```python
from build123d import *

# Parameters (mm, degrees)
SKETCH1_W             = 54
SKETCH1_H             = 54
BOSS_EXTRUDE1_DEPTH   = 10
CUT_EXTRUDE2_DEPTH    = 40.471508712
CUT_EXTRUDE3_DEPTH    = 2
SKETCH4_R             = 13.75
CUT_EXTRUDE4_DEPTH    = 1
SKETCH5_W             = 2
SKETCH5_H             = 10
SKETCH5_W_2           = 10
SKETCH5_H_2           = 2
CUT_EXTRUDE5_DEPTH    = 4
SKETCH7_R             = 8.75
CUT_EXTRUDE7_DEPTH    = 0.5
CROQUIS1_W            = 54
CROQUIS1_H            = 54
CORTAR_EXTRUIR1_DEPTH = 4


with BuildPart() as part:
    # Sketch1 → Boss-Extrude1 (new body)
    with BuildSketch(Plane(origin=(0, 0, 0), x_dir=(1, 0, 0), z_dir=(0, 1, 0))):
        Rectangle(SKETCH1_W, SKETCH1_H)
    extrude(amount=BOSS_EXTRUDE1_DEPTH)

    # Sketch2 → Cut-Extrude2 (cut, through all)
    with BuildSketch(Plane(origin=(0, 10, 0), x_dir=(1, 0, 0), z_dir=(0, 1, 0))):
        with BuildLine():
            ThreePointArc((-17, -14), (-16.121320344, -16.121320344), (-14, -17))
            Line((-14, -17), (-2, -17))
            Line((-2, -17), (-2, -14.866068747))
            ThreePointArc((-2, -14.866068747), (-10.606601718, -10.606601718), (-14.866068747, -2))
            Line((-14.866068747, -2), (-17, -2))
            Line((-17, -2), (-17, -14))
        make_face()
        with BuildLine():
            Line((2, -14.866068747), (2, -17))
            Line((2, -17), (14, -17))
            ThreePointArc((14, -17), (16.121320344, -16.121320344), (17, -14))
            Line((17, -14), (17, -2))
            Line((17, -2), (14.866068747, -2))
            ThreePointArc((14.866068747, -2), (10.606601718, -10.606601718), (2, -14.866068747))
        make_face()
        with BuildLine():
            Line((-17, 14), (-17, 2))
            Line((-17, 2), (-14.866068747, 2))
            ThreePointArc((-14.866068747, 2), (-10.606601718, 10.606601718), (-2, 14.866068747))
            Line((-2, 14.866068747), (-2, 17))
            Line((-2, 17), (-14, 17))
            ThreePointArc((-14, 17), (-16.121320344, 16.121320344), (-17, 14))
        make_face()
        with BuildLine():
            Line((14.866068747, 2), (17, 2))
            Line((17, 2), (17, 14))
            ThreePointArc((17, 14), (16.121320344, 16.121320344), (14, 17))
            Line((14, 17), (2, 17))
            Line((2, 17), (2, 14.866068747))
            ThreePointArc((2, 14.866068747), (10.606601718, 10.606601718), (14.866068747, 2))
        make_face()
    extrude(amount=-CUT_EXTRUDE2_DEPTH, mode=Mode.SUBTRACT)

    # Sketch3 → Cut-Extrude3 (cut)
    with BuildSketch(Plane(origin=(0, 10, 0), x_dir=(1, 0, 0), z_dir=(0, 1, 0))):
        with BuildLine():
            Line((-14, -17), (14, -17))
            ThreePointArc((14, -17), (16.121320344, -16.121320344), (17, -14))
            Line((17, -14), (17, 14))
            ThreePointArc((17, 14), (16.121320344, 16.121320344), (14, 17))
            Line((14, 17), (-14, 17))
            ThreePointArc((-14, 17), (-16.121320344, 16.121320344), (-17, 14))
            Line((-17, 14), (-17, -14))
            ThreePointArc((-17, -14), (-16.121320344, -16.121320344), (-14, -17))
        make_face()
    extrude(amount=-CUT_EXTRUDE3_DEPTH, mode=Mode.SUBTRACT)

    # Sketch4 → Cut-Extrude4 (cut)
    with BuildSketch(Plane(origin=(0, 8, 0), x_dir=(1, 0, 0), z_dir=(0, 1, 0))):
        with Locations(Location((0, 0, 0), (0, 0, 270))):
            Circle(SKETCH4_R)
    extrude(amount=-CUT_EXTRUDE4_DEPTH, mode=Mode.SUBTRACT)

    # Sketch5 → Cut-Extrude5 (cut)
    with BuildSketch(Plane(origin=(0, 10, 0), x_dir=(1, 0, 0), z_dir=(0, 1, 0))):
        with Locations((0, -22)):
            Rectangle(SKETCH5_W, SKETCH5_H)
        with BuildLine():
            Line((1, -17), (1, -13.713588152))
            ThreePointArc((1, -13.713588152), (0, -13.75), (-1, -13.713588152))
            Line((-1, -13.713588152), (-1, -17))
            Line((-1, -17), (1, -17))
        make_face()
        with Locations((22, 0)):
            Rectangle(SKETCH5_W_2, SKETCH5_H_2)
        with BuildLine():
            Line((17, 1), (13.713588152, 1))
            ThreePointArc((13.713588152, 1), (13.75, 0), (13.713588152, -1))
            Line((13.713588152, -1), (17, -1))
            Line((17, -1), (17, 1))
        make_face()
        with BuildLine():
            Line((1, 17), (-1, 17))
            Line((-1, 17), (-1, 13.713588152))
            ThreePointArc((-1, 13.713588152), (0, 13.75), (1, 13.713588152))
            Line((1, 13.713588152), (1, 17))
        make_face()
        with Locations((0, 22)):
            Rectangle(SKETCH5_W, SKETCH5_H)
        with Locations((-22, 0)):
            Rectangle(SKETCH5_W_2, SKETCH5_H_2)
        with BuildLine():
            Line((-13.713588152, 1), (-17, 1))
            Line((-17, 1), (-17, -1))
            Line((-17, -1), (-13.713588152, -1))
            ThreePointArc((-13.713588152, -1), (-13.75, 0), (-13.713588152, 1))
        make_face()
    extrude(amount=-CUT_EXTRUDE5_DEPTH, mode=Mode.SUBTRACT)

    # Sketch7 → Cut-Extrude7 (cut)
    with BuildSketch(Plane(origin=(0, 7, 0), x_dir=(1, 0, 0), z_dir=(0, 1, 0))):
        with Locations(Location((0, 0, 0), (0, 0, 270))):
            Circle(SKETCH7_R)
    extrude(amount=-CUT_EXTRUDE7_DEPTH, mode=Mode.SUBTRACT)

    # Croquis1 → Cortar-Extruir1 (cut)
    with BuildSketch(Plane.XZ):
        Rectangle(CROQUIS1_W, CROQUIS1_H)
    extrude(amount=-CORTAR_EXTRUIR1_DEPTH, mode=Mode.SUBTRACT)


solid = part.part
```
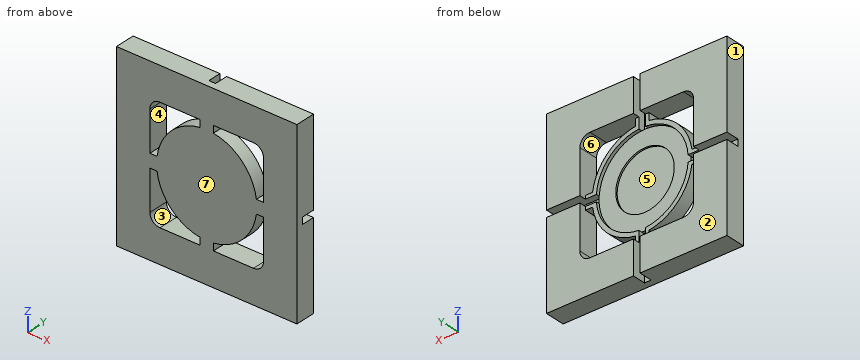
Build history of the part. All positions in model axes, mm. Face numbers are marked on the shaded views. A direction names the side the tool comes from. Round coordinates to 2 decimals unless told otherwise and drop trailing zeros. Order: outer loops, then holes, each group sorted by start corner. A loop starts at its lowest first (then second) coordinate and runs counter-clockwise, first axis right, second up. Notation, with made-up numbers: (-14.75, 40) -> (24.25, 40) arc R18 ccw to (24.25, 54) -> close; hole circle Ø7 at (47.25, -17.5). An arc over 180 degrees is marked (long way). Answer in a Markdown table with one row per item.
1) Mould opens along X. For the marked faces 1, 2, 3 and 4 say: released by +X, released by -X, zero draft, split by the parting line, or undercut.
Values:
| item | result |
|---|---|
| face 1 | released by -X |
| face 2 | zero draft |
| face 3 | undercut |
| face 4 | undercut |
2) Which spindle directions (+Z, -Z, +X, -X, +Y, -Y) get a long thin tool onto all of the face, cutting with end or side? Do the marked faces 5, 6 and 7. Say none if no direction does.
Values:
| item | result |
|---|---|
| face 5 | +Y |
| face 6 | +Y, -Y |
| face 7 | +Z, -Z, +X, -X, -Y |
3) Band-saw the part on D-D on z = 6.5. Give the cut face in (x, y).
Values:
| item | result |
|---|---|
| outline | (-27, 4) -> (-17, 4) -> (-17, 10) -> (-27, 10) -> close; (-13.52, 4) -> (13.52, 4) -> (13.52, 8) -> (12.12, 8) -> (12.12, 7) -> (5.86, 7) -> (5.86, 6.5) -> (-5.86, 6.5) -> (-5.86, 7) -> (-12.12, 7) -> (-12.12, 8) -> (-13.52, 8) -> close; (17, 4) -> (27, 4) -> (27, 10) -> (17, 10) -> close |
4) Band-saw the part on B-B on y = 9.1. Give the cut face in (x, z).
Values:
| item | result |
|---|---|
| outline | (-27, -27) -> (-1, -27) -> (-1, -17) -> (-14, -17) arc R3 cw to (-17, -14) -> (-17, -1) -> (-27, -1) -> close; (-27, 1) -> (-17, 1) -> (-17, 14) arc R3 cw to (-14, 17) -> (-1, 17) -> (-1, 27) -> (-27, 27) -> close; (1, -27) -> (27, -27) -> (27, -1) -> (17, -1) -> (17, -14) arc R3 cw to (14, -17) -> (1, -17) -> close; (1, 17) -> (14, 17) arc R3 cw to (17, 14) -> (17, 1) -> (27, 1) -> (27, 27) -> (1, 27) -> close |
5) Pin check, flat tips, straight feed: P1, Ø0.6, axis at x = 0, z = 21, coming from the +Y side; P2, Ø5, axis at x = -5.5, z = -6.5, coming from the +Y side; P3, Ø5, axis at x = -13, z = 13, coming from the +Y side. Stop position of each tip, or through.
Values:
| item | result |
|---|---|
| P1 | y = 6 |
| P2 | y = 7 |
| P3 | through |
6) Band-saw the part on A-A on z = 0. Give the cut face in (x, y), and give its area (3 significant figures).
Values:
| item | result |
|---|---|
| outline | (-27, 4) -> (27, 4) -> (27, 6) -> (13.75, 6) -> (13.75, 7) -> (8.75, 7) -> (8.75, 6.5) -> (-8.75, 6.5) -> (-8.75, 7) -> (-13.75, 7) -> (-13.75, 6) -> (-27, 6) -> close |
| area | 127 mm2 |
7) Band-saw the part on C-C on x = -10. Give the cut face in (y, z).
Values:
| item | result |
|---|---|
| outline | (4, -27) -> (10, -27) -> (10, -17) -> (4, -17) -> close; (4, -11.18) -> (8, -11.18) -> (8, -9.44) -> (7, -9.44) -> (7, 9.44) -> (8, 9.44) -> (8, 11.18) -> (4, 11.18) -> close; (4, 17) -> (10, 17) -> (10, 27) -> (4, 27) -> close |
8) Wall check: L1, parallel to X at y = 6.8, z = 0; L2, parallel to X at y = 8.8, z = 9.5. Give the ranges that are in metal, low to high.
Values:
| item | result |
|---|---|
| L1 | -13.75 to -8.75, 8.75 to 13.75 |
| L2 | -27 to -17, 17 to 27 |
